Build history of the part. All positions in model axes, mm. Face numbers are marked on the shaded views. A direction names the side the tool comes from. Coordinates: 2 decimals unless noted, no trailing zeros. Write each loop counter-clockwise with the first axis right and the second up, starting at its lowest first coordinate (ties: lowest second). Pieces come first, ordered by that corner, then holes.
from build123d import *


with BuildPart() as part:
    # Sketch1 → Revolve1 (revolve)
    with BuildSketch(Plane.YZ, mode=Mode.PRIVATE) as revolve1_sk:
        with BuildLine():
            Line((-107.334, 0), (-115.334, 0))
            Line((-115.334, 0), (-115.334, -12.1078633))
            ThreePointArc((-115.334, -12.1078633), (-115.891433721, -15.829164705), (-117.514800653, -19.22379227))
            Line((-117.514800653, -19.22379227), (-132.334, -41.130434783))
            Line((-132.334, -41.130434783), (-132.334, -50))
            Line((-132.334, -50), (-130.334, -50))
            Line((-130.334, -50), (-107.334, -16))
            Line((-107.334, -16), (-15.875, -16))
            Line((-15.875, -16), (-15.875, -8))
            Line((-15.875, -8), (-10, -8))
            Line((-10, -8), (-10, -5))
            Line((-10, -5), (-40, -5))
            Line((-40, -5), (-40, -3.333333333))
            Line((-40, -3.333333333), (-70, -3.333333333))
            Line((-70, -3.333333333), (-70, -1.666666667))
            Line((-70, -1.666666667), (-107.334, -1.666666667))
            Line((-107.334, -1.666666667), (-107.334, 0))
        make_face()
    revolve(revolve1_sk.sketch.rotate(Axis((0, 0, 55), (0, 0, -1)), 270), axis=Axis((0, 0, 55), (0, 0, -1)))


solid = part.part
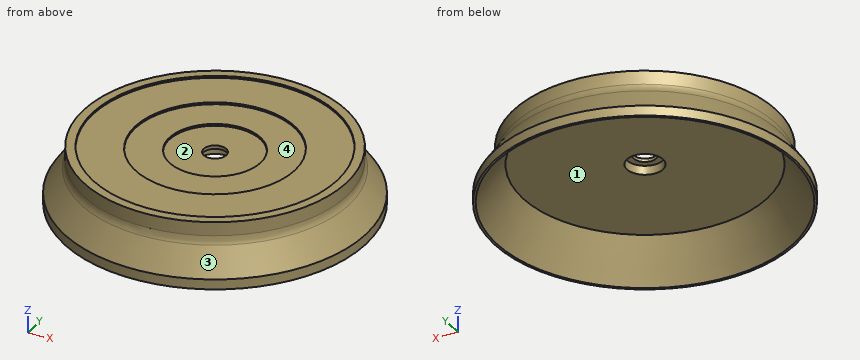
(1) Slice it at D-D, the plane z = -36.5. List the corners of the cut face in (x, y), and give its area (3 significant figures).
(2) Two-plate mould, pull along Y, no slides. Class the marked faces 3 and 4: pulls with the +Y half, pulls with the -Y half, needs draft (parallel to the pull), parting line crosses it, or undercut.
(3) 3-axis set-ups, long thin cutter, end or side, ignore diameter. For the marked faces 1 and 2: which of +Z, -Z, +X, -X, +Y, -Y reach the whole face in a straight line?
(4) Slice it at C-C, the plane z = -22.5. List the corners of the cut face in (x, y), and give its area (3 significant figures).
(5) Probe L1, parallel to Y at x = 0, z = -4.4; L2, parallel to Y at x = 0, z = -1; L3, parallel to Z at x = 13, y = 71. List the from-to ranges inside material, lowest first.
(6) Flat gauge pins, fed straight in: P1, Ø10, axis at y = 82.5, z = -10, coming from the +X side; P2, Ø4, axis at x = -80, y = -44.5, coming from the -Z side; P3, Ø10, axis at y = -62.5, z = -14.5, coming from the -X side. Where does each tip first touch, or does it go through?
Results:
1. outline: circle Ø258.4 at (0, 0); hole circle Ø242.4 at (0, 0)
1. area: 6,290 mm2
2. face 3: parting line crosses it
2. face 4: undercut
3. face 1: -Z
3. face 2: +Z
4. outline: circle Ø239.46 at (0, 0); hole circle Ø223.46 at (0, 0)
4. area: 5,820 mm2
5. L1: y = -115.33 to -40, 40 to 115.33
5. L2: y = -115.33 to -107.33, 107.33 to 115.33
5. L3: z = -16 to -1.67
6. P1: stops at x = 85.41
6. P2: stops at z = -16
6. P3: stops at x = -100.83
